from build123d import *

# Parameters (mm, degrees)
SKETCH1_R                = 9.54278
BOSS_EXTRUDE1_DEPTH      = 25.4
SKETCH2_R                = 12.7
BOSS_EXTRUDE2_DEPTH      = 6.35
R_0_339_DIAMETER_HOLE1_D = 8.6106


with BuildPart() as part:
    # Sketch1 → Boss-Extrude1 (new body)
    with BuildSketch(Plane(origin=(0, 0, 0), x_dir=(1, 0, 0), z_dir=(0, 1, 0))):
        with Locations(Location((0, 0, 0), (0, 0, 270))):
            Circle(SKETCH1_R)
    extrude(amount=BOSS_EXTRUDE1_DEPTH)

    # Sketch2 → Boss-Extrude2 (add)
    with BuildSketch(Plane(origin=(0, 25.4, 0), x_dir=(1, 0, 0), z_dir=(0, 1, 0))):
        with Locations(Location((0, 0, 0), (0, 0, 270))):
            Circle(SKETCH2_R)
    extrude(amount=-BOSS_EXTRUDE2_DEPTH)

    # R (0.339) Diameter Hole1 (through all)
    with Locations(Plane(origin=(0, 25.4, 0), x_dir=(1, 0, 0), z_dir=(0, 1, 0))):
        with Locations((0, 0)):
            Hole(R_0_339_DIAMETER_HOLE1_D / 2)

    # Sketch4 → 1/8 NPT Tapped Hole1 (revolve, cut)
    with BuildSketch(Plane(origin=(0, 25.4, 0), x_dir=(0, 0, 1), z_dir=(1, 0, 0))):
        Polygon((0, 0), (0, 14.478), (4.2164, 11.944531286), (4.2164, 9.652), (4.537399894, 9.652), (4.8263937, 0), align=None)
    revolve(axis=Axis((0, 31.75, 0), (0, -1, 0)), mode=Mode.SUBTRACT)

    # Sketch6 → 1/8 NPT Tapped Hole2 (revolve, cut)
    with BuildSketch(Plane(origin=(0, 0, 0), x_dir=(0, 0, -1), z_dir=(1, 0, 0))):
        Polygon((0, 0), (0, 14.478), (4.2164, 11.944531286), (4.2164, 9.652), (4.537399894, 9.652), (4.8263937, 0), align=None)
    revolve(axis=Axis((0, -6.35, 0), (0, 1, 0)), mode=Mode.SUBTRACT)

    # Sketch9 → Cut-Revolve1 (revolve, cut)
    with BuildSketch(Plane(origin=(0, 0, 0), x_dir=(0, 0, -1), z_dir=(1, 0, 0))):
        Polygon((-9.314991403, 0), (-9.54278, 13.05), (-9.54278, 0), align=None)
    revolve(axis=Axis((0, 19.05, 0), (0, -1, 0)), mode=Mode.SUBTRACT)


solid = part.part
The model under review builds one solid part; all positions refer to its coordinate system, in mm. A direction names the side the tool comes from. Give positions to 0.01 mm unless a question says otherwise; leave off trailing zeros. Write each loop counter-clockwise with the first axis right and the second up, starting at its lowest first coordinate (ties: lowest second). Pieces come first, ordered by that corner, then holes.
1. Add section A-A, the plane y = 5.5. Write out the cut boundary in (x, z), plus the area to 3 significant figures.
2. Add section C-C, the plane x = 10.5. Write out the cut boundary in (y, z), plus the area to 3 significant figures.
3. Tool access review of faces 5 (the cylindrical face through (-5.81, 16.01, -7.57)), 6 (the flat face through (0, 25.4, 5)): name each direction out of +Z, -Z, +X, -X, +Y, -Y from which nothing blocks a thin tool from reaching the whole face with its end or side.
4. For P1, Ø4, axis at x = -9.5, y = 22.5, coming from the -Z side; P2, Ø1, axis at x = -7.5, y = 21.5, coming from the +Z side; P3, Ø5, axis at y = 6.5, z = 5.5, coming from the -X side, all flat-tipped, find the tip position at first contact; note any pin that passes through.
5. Draft analysis for pull direction X (two halves, no side actions). For faces 1 (the conical face through (-4.644, 4.758, 0.61)), 2 (the conical face through (-4.644, 20.642, -0.61)), 3 (the conical face through (-2.833, 6.616, 8.995)), 4 (the flat face through (-4, 0, 4)), state which applies: +X half, -X half, draft (parallel to the pull), parting line (faces both ways), or undercut.
6. Add section D-D, the plane y = 20. Write out the cut boundary in (x, z).
7. Add section B-B, the plane z = 10.5. Write out the cut boundary in (x, y).
8. Wall thickness on L1, parallel to Z at x = 0, y = 14.5; L2, parallel to Y at x = -5.5, z = 9.25; L3, parallel to Y at x = 1.5, z = 4.25: over which ranges is each line inside the solid? List them lowest first.
Worked answers:
1. outline: circle Ø18.82 at (0, 0); hole circle Ø9.32 at (0, 0)
1. area: 210 mm2
2. outline: (19.05, -7.14) - (25.4, -7.14) - (25.4, 7.14) - (19.05, 7.14) - close
2. area: 90.7 mm2
3. face 5: -Y
3. face 6: +Z, -Z, +X, -X, +Y
4. P1: stops at z = -10.25
4. P2: stops at z = 10.6
4. P3: stops at x = -8.94
5. face 1: undercut
5. face 2: undercut
5. face 3: parting line
5. face 4: draft
6. outline: circle Ø25.4 at (0, 0); hole circle Ø9.33 at (0, 0)
7. outline: (-7.14, 19.05) - (7.14, 19.05) - (7.14, 25.4) - (-7.14, 25.4) - close
8. L1: z = -9.54 to -4.31, 4.31 to 9.54
8. L2: y = 19.05 to 25.4
8. L3: y = 9.65 to 15.75
